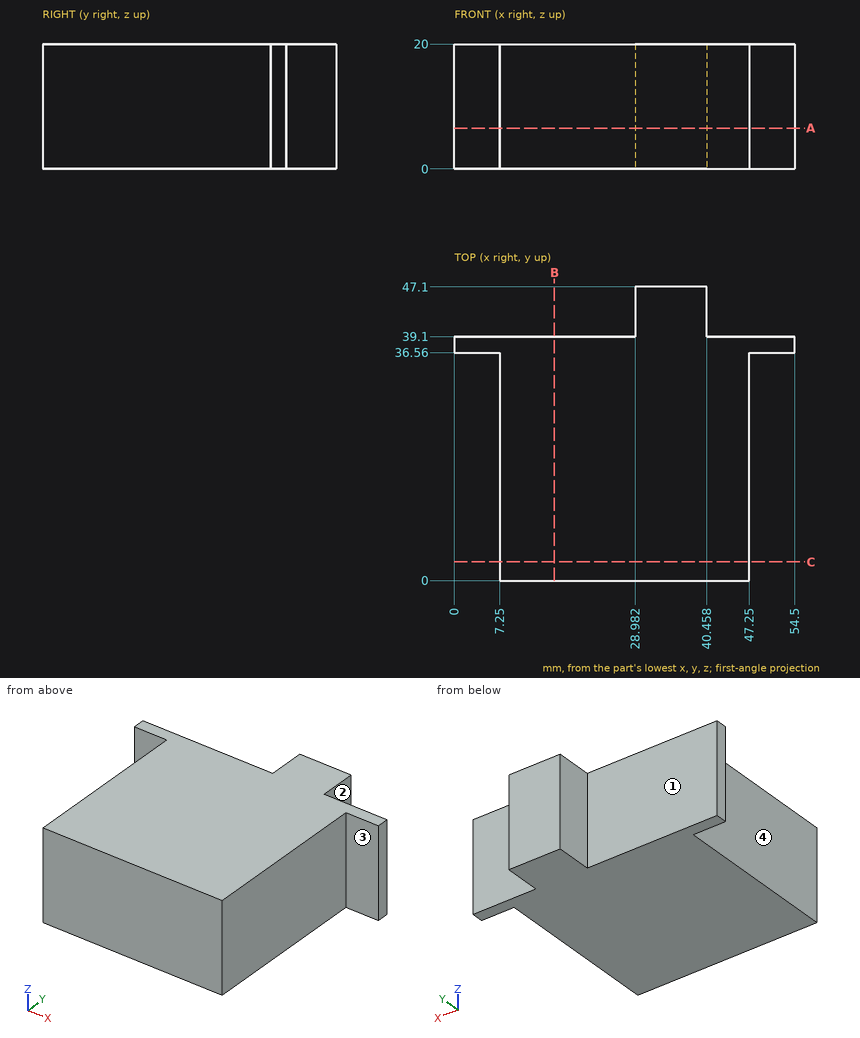
Print and shaded views of the part. All mm, measured from the part's lowest x, y and z. A direction names the side the tool comes from. Coordinates: 2 decimals unless noted, no trailing zeros. Write each loop counter-clockwise with the first axis right and the second up, starting at its lowest first coordinate (ties: lowest second). Pieces come first, ordered by that corner, then holes.
(1) Drill centre lines: probe 1 along X at (y, z) = (27, 16); probe 2 along Y at (x, z) = (11, 7.75); probe 3 along Y at (x, z) = (7, 11.75). Where is each one in solid material? Low to high.
(2) Cut at B-B, the plane x = 16. List the corners of the cut face in (y, z), and give its area (3 significant figures).
(3) Cut at A-A, the plane z = 6.5. List the corners of the cut face in (x, y).
(4) 3-axis set-ups, long thin cutter, end or side, ignore diameter. For the marked faces 1, 2, 3 and 4: which of +Z, -Z, +X, -X, +Y, -Y reach the whole face in a straight line?
(5) Flat gauge pins, fed straight in: pin 1 (8 mm diameter, centred on x = 2.5, z = 12, fed in from -Y); pin 2 (2.5 mm diameter, centred on y = 42, z = 11.5, fed in from +X); pin 3 (2.5 mm diameter, centred on y = 44, z = 10.5, fed in from -X). Where does each tip first touch, or does it go through?
(6) Cut at C-C, the plane y = 3. List the corners of the cut face in (x, z), and give its area (3 significant figures).
Geometry says:
1. probe 1: x = 7.25 to 47.25
1. probe 2: y = 0 to 39.1
1. probe 3: y = 36.56 to 39.1
2. outline: (0, 0) - (39.1, 0) - (39.1, 20) - (0, 20) - close
2. area: 782 mm2
3. outline: (0, 36.56) - (7.25, 36.56) - (7.25, 0) - (47.25, 0) - (47.25, 36.56) - (54.5, 36.56) - (54.5, 39.1) - (40.46, 39.1) - (40.46, 47.1) - (28.98, 47.1) - (28.98, 39.1) - (0, 39.1) - close
4. face 1: +Z, -Z, -X, +Y
4. face 2: +Z, -Z, +X, +Y
4. face 3: +Z, -Z, +X, -Y
4. face 4: +Z, -Z, -X, -Y
5. pin 1: stops at y = 36.56
5. pin 2: stops at x = 40.46
5. pin 3: stops at x = 28.98
6. outline: (7.25, 0) - (47.25, 0) - (47.25, 20) - (7.25, 20) - close
6. area: 800 mm2
